Geometry check sheet. Reference: the model listing, model coordinates, mm. A direction names the side the tool comes from. Round coordinates to 2 decimals unless told otherwise and drop trailing zeros. Loops run counter-clockwise (first coordinate to the right, second up) from the corner with the lowest first, then second, coordinate; pieces in that order, holes last.
Autodesk Inventor part; units mm, degrees
ref_plane "YZ Plane" through (0, 0, 0) normal (1, 0, 0) x (0, 1, 0)
ref_plane "XZ Plane" through (0, 0, 0) normal (0, 1, 0) x (-1, 0, 0)
ref_plane "XY Plane" through (0, 0, 0) normal (0, 0, 1) x (1, 0, 0)
sketch "Sketch1" plane through (0, 0, 0) normal (0, 1, 0) x (-1, 0, 0)
  point P0 (0, 0)
sketch "Sketch2" plane through (0, 0, 0) normal (0, 1, 0) x (-1, 0, 0)
  line L0 (0, 0) -> (0, -147)
  line L1 (0, -147) -> (78, -147)
  line L2 (78, -147) -> (78, 0)
  line L3 (78, 0) -> (0, 0)
  dimension "d0" = 147
  dimension "d1" = 78
extrude "Extrusion1" add sketch "Sketch2" along normal blind 5
sketch "Sketch3" plane through (0, 5, 0) normal (0, 1, 0) x (1, 0, 0)
  line L0 (0, 0) -> (0, 147)
  line L1 (-78, 0) -> (0, 0)
  line L2 (0, 0) -> (-4, 0)
  line L3 (-4, 0) -> (-4, 66)
  line L4 (-4, 66) -> (0, 66)
  dimension "d4" = 4
  dimension "d5" = 66
extrude "Extrusion2" add sketch "Sketch3" along normal blind 35
sketch "Sketch4" plane through (0, 5, 0) normal (0, 1, 0) x (1, 0, 0)
  line L0 (-4, 66) -> (0, 66)
  line L1 (0, 66) -> (0, 147)
  line L2 (0, 66) -> (0, 79)
  line L3 (0, 79) -> (-4, 79)
  line L4 (-4, 79) -> (-4, 66)
  point P0 (0, 0)
  dimension "d8" = 13
extrude "Extrusion3" add sketch "Sketch4" along normal blind 28
sketch "Sketch5" plane through (0, 5, 0) normal (0, 1, 0) x (1, 0, 0)
  line L0 (-4, 79) -> (0, 79)
  line L1 (0, 79) -> (0, 147)
  line L2 (0, 147) -> (-78, 147)
  line L3 (-4, 79) -> (-4, 147)
  line L4 (0, 147) -> (0, 79)
  point P0 (0, 0)
extrude "Extrusion4" add sketch "Sketch5" along normal blind 35
sketch "Sketch6" plane through (0, 5, 0) normal (0, 1, 0) x (1, 0, 0)
  line L0 (-4, 0) -> (-4, 147)
  line L1 (-4, 147) -> (-78, 147)
  line L2 (-78, 147) -> (-78, 0)
  line L3 (-4, 147) -> (-4, 141)
  line L4 (-4, 141) -> (-78, 141)
  line L5 (-78, 147) -> (-4, 147)
  point P0 (0, 0)
  dimension "d13" = 6
extrude "Extrusion5" add sketch "Sketch6" along normal blind 35
sketch "Sketch7" plane through (0, 5, 0) normal (0, 1, 0) x (1, 0, 0)
  line L0 (-4, 141) -> (-78, 141)
  line L1 (-78, 141) -> (-78, 0)
  line L2 (-78, 0) -> (-4, 0)
  line L3 (-78, 141) -> (-78, 0)
  line L4 (-78, 0) -> (-70, 0)
  line L5 (-70, 0) -> (-70, 141)
  point P0 (0, 0)
  dimension "d16" = 8
extrude "Extrusion6" add sketch "Sketch7" along normal blind 35
sketch "Sketch8" plane through (0, 5, 0) normal (0, 1, 0) x (1, 0, 0)
  line L0 (-70, 141) -> (-70, 0)
  line L1 (-70, 0) -> (-4, 0)
  line L2 (-4, 0) -> (-4, 141)
  line L3 (-4, 141) -> (-70, 141)
  line L4 (-4, 0) -> (-70, 0)
  line L5 (-4, 0) -> (-4, 6)
  line L6 (-4, 6) -> (-70, 6)
  point P0 (0, 0)
  dimension "d19" = 6
extrude "Extrusion7" add sketch "Sketch8" along normal blind 35 contours L6 L2 L1 L0
properties part number "caixav2"
1) Mould release check, pull along X, two halves, no side actions. Record for faces 4 (the face through (0, 20, -72)), 5 (the face through (-37, 22, -141)), 6 (the face through (-2, 36, -66)): +X half, -X half, draft (parallel to the pull), parting line (faces both ways), or undercut.
Report:
face 4: +X half
face 5: undercut
face 6: draft
2) Sectioned sample at C-C, the plane z = -69.5. Record the cut outline in (x, y), then the cut area to 3 significant figures.
Report:
outline: (-78, 0) - (0, 0) - (0, 33) - (-4, 33) - (-4, 5) - (-70, 5) - (-70, 40) - (-78, 40) - close
area: 782 mm2
3) Scan lines: line 1 along X through (y, z) = (11, -84.5); line 2 along Z through (x, y) = (-18, 37.5); line 3 along Y through (x, z) = (-43.5, -115). Record each from-to range of solid material in increasing order.
Report:
line 1: x = -78 to -70, -4 to 0
line 2: z = -147 to -141, -6 to 0
line 3: y = 0 to 5
4) Access from +Z, -Z, +X, -X, +Y, -Y to the whole of each face (thin tool, end or side, straight path). Record for faces 1 (the face through (-2, 33, -73)), 2 (the face through (-4, 22, -73)), 3 (the face through (-40, 20, 0)).
Report:
face 1: +X, +Y
face 2: +Y
face 3: +Z, +X, -X, +Y, -Y
5) Sectioned sample at A-A, the plane y = 25.5. Record the cut outline in (x, z).
Report:
outline: (-78, -147) - (0, -147) - (0, 0) - (-78, 0) - close; hole (-70, -141) - (-4, -141) - (-4, -6) - (-70, -6) - close
6) Gauge pin test, flat ends, axial feed: pin 1 (2 mm diameter, centred on x = -16.5, z = -15, fed in from +Y); pin 2 (1.2 mm diameter, centred on x = -2, z = -72.5, fed in from +Y). Record the tip position at first contact, or that the pin passes through.
Report:
pin 1: stops at y = 5
pin 2: stops at y = 33
7) Sectioned sample at D-D, the plane y = 34.5. Record the cut outline in (x, z).
Report:
outline: (-78, -147) - (0, -147) - (0, -79) - (-4, -79) - (-4, -141) - (-70, -141) - (-70, -6) - (-4, -6) - (-4, -66) - (0, -66) - (0, 0) - (-78, 0) - close
8) Sectioned sample at B-B, the plane x = -13. Record the cut outline in (y, z), then the cut area to 4 significant figures.
Report:
outline: (0, -147) - (40, -147) - (40, -141) - (5, -141) - (5, -6) - (40, -6) - (40, 0) - (0, 0) - close
area: 1,155 mm2
